```python
from build123d import *

# Parameters (mm, degrees)
BOSS_EXTRUDE1_DEPTH = 6
FILLET1_R           = 2
BOSS_EXTRUDE2_DEPTH = 10
FILLET2_R           = 2


with BuildPart() as part:
    # Sketch1 → Boss-Extrude1 (new body)
    with BuildSketch(Plane.XY):
        Polygon((-16.461538462, -8.743589744), (-8.461538462, -8.743589744), (-8.461538462, -5.743589744), (4.538461538, -5.743589744), (4.538461538, -8.743589744), (12.538461538, -8.743589744), (12.538461538, -4.743589744), (8.538461538, -4.743589744), (8.538461538, -1.743589744), (-12.461538462, -1.743589744), (-12.461538462, -4.743589744), (-16.461538462, -4.743589744), align=None)
    extrude(amount=BOSS_EXTRUDE1_DEPTH)

    # Fillet1
    fillet1_edges = [part.edges().sort_by_distance(p)[0] for p in [
        (-16.461538462, -4.743589744, 3),
        (-12.461538462, -1.743589744, 3),
        (8.538461538, -1.743589744, 3),
        (12.538461538, -4.743589744, 3),
    ]]
    fillet(fillet1_edges, radius=FILLET1_R)

    # Sketch3 → Boss-Extrude2 (add)
    with BuildSketch(Plane.XY.offset(6)):
        Polygon((-8.461538462, -5.743589744), (-8.461538462, -8.743589744), (-12.461538462, -8.743589744), (-12.461538462, -4.743589744), (-12.461538462, -1.743589744), (-10.461538462, -1.743589744), (8.538461538, -1.743589744), (8.538461538, -4.743589744), (8.538461538, -8.743589744), (4.538461538, -8.743589744), (4.538461538, -5.743589744), align=None)
    extrude(amount=BOSS_EXTRUDE2_DEPTH)

    # Fillet2
    fillet2_edges = [part.edges().sort_by_distance(p)[0] for p in [
        (8.538461538, -1.743589744, 11),
        (-12.461538462, -1.743589744, 11),
    ]]
    fillet(fillet2_edges, radius=FILLET2_R)


solid = part.part
```
The listing builds one solid part. Answer for the finished solid, in the listing's coordinates (mm). A direction names the side the tool comes from. Coordinates: 2 decimals unless noted, no trailing zeros. Write each loop counter-clockwise with the first axis right and the second up, starting at its lowest first coordinate (ties: lowest second). Pieces come first, ordered by that corner, then holes. Notation, with made-up numbers: (-33.5, -5.5) - (-11.5, -5.5) arc R25 ccw to (-11.5, 11.5) - close; hole circle Ø2 at (-31.75, 0). An arc over 180 degrees is marked (long way). Return JSON: item names as keys, results as strings. Group by question number.
Q1. The part is cut by section D-D on y = -2.25. Write down the section's boundary in (x, z), and give its area (3 significant figures).
Q2. The part is cut by section B-B on x = 3. Write down the section's boundary in (y, z), and give its area (3 significant figures).
Q3. The part is cut by section A-A on z = 4.5. Write down the section's boundary in (x, y), and give its area (3 significant figures).
Q4. Which of the six approach directions +Z, -Z, +X, -X, +Y, -Y give full straight-line access (tool end or side, diameter ignored) to faces 1 (the cylindrical face through (7.968, -2.345, 3.042)), 2 (the flat face through (-14, -7, 6)), 3 (the flat face through (-12, -8.744, 6)), 4 (the flat face through (-13, -4.744, 3)), 5 (the flat face through (4.538, -7, 8))?
Q5. The part is cut by section C-C on z = 12.5. Write down the section's boundary in (x, y), and give its area (3 significant figures).
Q6. Find the intervals of material crossed by line 1 along X through (y, z) = (-8.5, 5.25); line 2 along X through (y, z) = (-6.75, 11.5); line 3 along Y through (x, z) = (-4.5, 2.25), in increasing order. Write a range as [from, to].
Q7. Flat-ended cylindrical pins translate along their axes: pin 1 Ø4 at (x, z) = (-1.5, 4.5) entering from -Y; pin 2 Ø1 at (x, y) = (-11, -2.5) entering from -Z; pin 3 Ø2.5 at (y, z) = (-6, 8) entering from +X; pin 4 Ø3 at (y, z) = (-6, 11.5) entering from -X. Find the tip coordinate at first contact, or state that the pin passes through.
Evaluation:
{
 "1": {"outline": "(-11.79, 0) - (7.87, 0) - (7.87, 16) - (-11.79, 16) - close", "area": "315 mm2"},
 "2": {"outline": "(-5.74, 0) - (-1.74, 0) - (-1.74, 16) - (-5.74, 16) - close", "area": "64.0 mm2"},
 "3": {"outline": "(-16.46, -8.74) - (-8.46, -8.74) - (-8.46, -5.74) - (4.54, -5.74) - (4.54, -8.74) - (12.54, -8.74) - (12.54, -6.74) arc R2 ccw to (10.54, -4.74) - (8.54, -4.74) - (8.54, -3.74) arc R2 ccw to (6.54, -1.74) - (-10.46, -1.74) arc R2 ccw to (-12.46, -3.74) - (-12.46, -4.74) - (-14.46, -4.74) arc R2 ccw to (-16.46, -6.74) - close", "area": "137 mm2"},
 "4": {"face 1": "+Z, -Z, +X, +Y", "face 2": "+Z, -X, +Y, -Y", "face 3": "+Z, -Z, +X, -X, -Y", "face 4": "+Z, -Z, -X, +Y", "face 5": "+Z, -Z, -Y"},
 "5": {"outline": "(-12.46, -8.74) - (-8.46, -8.74) - (-8.46, -5.74) - (4.54, -5.74) - (4.54, -8.74) - (8.54, -8.74) - (8.54, -3.74) arc R2 ccw to (6.54, -1.74) - (-10.46, -1.74) arc R2 ccw to (-12.46, -3.74) - close", "area": "106 mm2"},
 "6": {"line 1": "x = [-16.46, -8.46], [4.54, 12.54]", "line 2": "x = [-12.46, -8.46], [4.54, 8.54]", "line 3": "y = [-5.74, -1.74]"},
 "7": {"pin 1": "stops at y = -5.74", "pin 2": "stops at z = 0", "pin 3": "stops at x = 8.54", "pin 4": "stops at x = -12.46"}
}
